The model under review builds one solid part; all positions refer to its coordinate system, in mm. Face numbers are marked on the shaded views. A direction names the side the tool comes from. Round coordinates to 2 decimals unless told otherwise and drop trailing zeros. Loops run counter-clockwise (first coordinate to the right, second up) from the corner with the lowest first, then second, coordinate; pieces in that order, holes last. Notation, with made-up numbers: (70, 76.25) -> (78, 76.25) arc R11 cw to (78, 93.25) -> close; hole circle Ø9 at (66, 5). An arc over 180 degrees is marked (long way). Use a Markdown table: item, result. Add a question column.
1) Insertion check: pin 1 (1 mm diameter, centred on x = -3.5, y = 6, fed in from +Z); pin 2 (2 mm diameter, centred on x = -4, z = -3.5, fed in from -Y); pin 3 (1 mm diameter, centred on x = -3.5, y = 6, fed in from -Z); pin 4 (3.5 mm diameter, centred on x = 3.62, z = 0, fed in from +Y). Each pin has a flat end and moves straight along its axis. Give the tip position at first contact, or say it passes through.
2) For the marked faces 4, 5 and 6, list the 3-axis set-ups (+Z, -Z, +X, -X, +Y, -Y) from which the entire face can be reached by the end or side of a thin tool; tool diameter is ignored.
3) Consider section A-A on x = 0. Give the boundary of the cut face in (y, z) (3 decimals).
4) Wall thickness on probe 1 along Z at (x, y) = (4, 1.75); probe 2 along Z at (x, y) = (3.75, 5.75); probe 3 along Y at (x, z) = (-2, 4.5): over which ranges is each line inside the solid? List them lowest first.
5) Mouldability with a two-part tool opening along Z and no side actions: class the marked faces 1, 2 and 3 as released by +Z, released by -Z, zero draft, split by the parting line, or undercut.
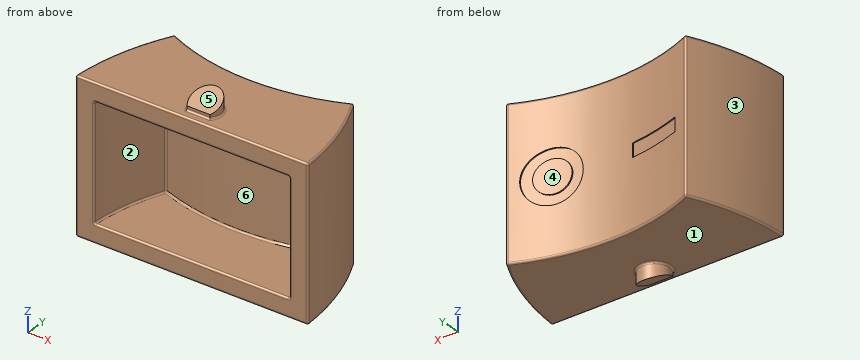
from build123d import *

# Parameters (mm, degrees)
BOSS_EXTRUDE1_DEPTH     = 5.207
SHELL1_T                = -1.27
BOSS_EXTRUDE2_REACH     = 16.757
CUT_EXTRUDE1_REACH      = 39.593
CUT_EXTRUDE1_END_RADIUS = 14.8082
CUT_EXTRUDE1_START      = -25.4
SKETCH11_R              = 1.8415
SKETCH11_R_2            = 1.143
SKETCH11_W              = 3.556
SKETCH11_H              = 0.9525
FILLET1_R               = 0.127


with BuildPart() as part:
    # Sketch1 → Boss-Extrude1 (new, symmetric)
    with BuildSketch(Plane(origin=(0, 0, 0), x_dir=(-1, 0, 0), z_dir=(0, 0, -1))):
        with BuildLine():
            Line((-8.001, 0), (8.001, 0))
            ThreePointArc((8.001, 0), (7.451075327, 3.466952212), (6.1595, 6.731))
            ThreePointArc((6.1595, 6.731), (0, 5.381540258), (-6.1595, 6.731))
            ThreePointArc((-6.1595, 6.731), (-7.451075327, 3.466952212), (-8.001, 0))
        make_face()
    extrude(amount=BOSS_EXTRUDE1_DEPTH, both=True)

    # Shell1
    shell1_openings = [part.faces().sort_by_distance(p)[0] for p in [
        (0, 0, 0),
    ]]
    offset(amount=SHELL1_T, openings=shell1_openings, kind=Kind.INTERSECTION)

    # Boss-Extrude2: up to this plane
    boss_extrude2_end = Plane(origin=(0, -1.994396708, 4.276997542), z_dir=(0, -0.4226182617407003, 0.9063077870366496))
    # Sketch5 → Boss-Extrude2 (add, up to the surface)
    with BuildSketch(Plane.XY.offset(5.207), mode=Mode.PRIVATE) as boss_extrude2_sk1:
        with BuildLine():
            Line((0.793114746, 0.635), (-0.793114746, 0.635))
            ThreePointArc((-0.793114746, 0.635), (0, 2.286), (0.793114746, 0.635))
        make_face()
    boss_extrude2_tool1 = split(extrude(boss_extrude2_sk1.sketch, amount=BOSS_EXTRUDE2_REACH, mode=Mode.PRIVATE), bisect_by=boss_extrude2_end, keep=Keep.BOTH, mode=Mode.PRIVATE)
    boss_extrude2 = boss_extrude2_tool1.solids().sort_by_distance((0, 1.387858, 5.207))[0]
    add(boss_extrude2)

    # Mirror2: Boss-Extrude2 across plane
    add(boss_extrude2.mirror(Plane.XY))

    # Cut-Extrude1: up to this cylinder (the profile starts inside it)
    cut_extrude1_end = Plane(origin=(0, 20.113540258, 0), z_dir=(0, 0, -1)) * Cylinder(CUT_EXTRUDE1_END_RADIUS, 109.8024, mode=Mode.PRIVATE)
    # Sketch11 → Cut-Extrude1 (cut, up to the surface)
    with BuildSketch(Plane.XZ.offset(CUT_EXTRUDE1_START), mode=Mode.PRIVATE) as cut_extrude1_sk1:
        with Locations(Location((3.6195, 0, 0), (0, 0, 180))):
            Circle(SKETCH11_R)
        with Locations(Location((3.6195, 0, 0), (0, 0, 180))):
            Circle(SKETCH11_R_2, mode=Mode.SUBTRACT)
    cut_extrude1_tool1 = extrude(cut_extrude1_sk1.sketch, amount=CUT_EXTRUDE1_REACH, mode=Mode.PRIVATE) & cut_extrude1_end
    add(cut_extrude1_tool1.solids().sort_by_distance((5.408915, 25.4, 0))[0], mode=Mode.SUBTRACT)
    # Sketch11 → Cut-Extrude1 (cut, up to the surface)
    with BuildSketch(Plane.XZ.offset(CUT_EXTRUDE1_START), mode=Mode.PRIVATE) as cut_extrude1_sk2:
        with Locations((-3.3655, 0)):
            Rectangle(SKETCH11_W, SKETCH11_H)
    cut_extrude1_tool2 = extrude(cut_extrude1_sk2.sketch, amount=CUT_EXTRUDE1_REACH, mode=Mode.PRIVATE) & cut_extrude1_end
    add(cut_extrude1_tool2.solids().sort_by_distance((-3.3655, 25.4, 0))[0], mode=Mode.SUBTRACT)

    # Fillet1
    fillet1_edges = [part.edges().sort_by_distance(p)[0] for p in [
        (0, 0, 5.207),
        (-7.451075327, 3.466952212, 5.207),
        (0, 4.111540258, 3.937),
        (5.535048759, 5.099305704, 0),
        (-6.360295192, 2.603068492, 3.937),
        (-5.535048759, 5.099305704, 0),
        (0, 0, 3.937),
        (-6.729437878, 0, 0),
        (6.360295192, 2.603068492, 3.937),
        (6.729437878, 0, 0),
        (0, 4.111540258, -3.937),
        (6.360295192, 2.603068492, -3.937),
        (0, 0, -3.937),
        (-6.360295192, 2.603068492, -3.937),
        (0, 2.286, 5.207),
        (0, 0.635, 5.207),
        (0, 2.286, -5.207),
        (0, 0.635, -5.207),
        (0, 5.381540258, 5.207),
        (-7.451075327, 3.466952212, -5.207),
        (0, 0, -5.207),
        (7.451075327, 3.466952212, -5.207),
        (0, 5.381540258, -5.207),
        (7.451075327, 3.466952212, 5.207),
        (-6.1595, 6.731, 0),
        (-8.001, 0, 0),
        (8.001, 0, 0),
        (6.1595, 6.731, 0),
    ]]
    fillet(fillet1_edges, radius=FILLET1_R)


solid = part.part
Result set:
| question | item | result |
|---|---|---|
| 1 | pin 1 | z = 5.21 |
| 1 | pin 2 | y = 0 |
| 1 | pin 3 | z = -5.21 |
| 1 | pin 4 | y = 6.31 |
| 2 | face 4 | +Z, -Z, +Y |
| 2 | face 5 | +Z, +X, -X, -Y |
| 2 | face 6 | -Y |
| 3 | outline | (0, -5.08) arc R0.127 ccw to (0.127, -5.207) -> (0.508, -5.207) arc R0.127 cw to (0.635, -5.334) -> (0.635, -5.503) -> (2.286, -6.273) -> (2.286, -5.334) arc R0.127 cw to (2.413, -5.207) -> (5.255, -5.207) arc R0.127 ccw to (5.382, -5.08) -> (5.382, 5.08) arc R0.127 ccw to (5.255, 5.207) -> (2.413, 5.207) arc R0.127 cw to (2.286, 5.334) -> (2.286, 6.273) -> (0.635, 5.503) -> (0.635, 5.334) arc R0.127 cw to (0.508, 5.207) -> (0.127, 5.207) arc R0.127 ccw to (0, 5.08) -> (0, 4.064) arc R0.127 ccw to (0.127, 3.937) -> (3.985, 3.937) arc R0.127 cw to (4.112, 3.81) -> (4.112, -3.81) arc R0.127 cw to (3.985, -3.937) -> (0.127, -3.937) arc R0.127 ccw to (0, -4.064) -> close |
| 4 | probe 1 | -5.21 to -3.94, 3.94 to 5.21 |
| 4 | probe 2 | -5.21 to 5.21 |
| 4 | probe 3 | 0 to 5.52 |
| 5 | face 1 | released by -Z |
| 5 | face 2 | undercut |
| 5 | face 3 | zero draft |
